Can you work these out from the model? Positions are in its coordinate system, mm. A direction names the side the tool comes from. Coordinates: 2 decimals unless noted, no trailing zeros. Write each loop counter-clockwise with the first axis right and the second up, starting at its lowest first coordinate (ties: lowest second). Pieces come first, ordered by that corner, then holes. Notation, with made-up numbers: M -12.75,-23 L 6.25,-23 A23 cw 6.25,5 Z; hole C 18,86.25 d5. An arc over 180 degrees is marked long. Answer as a JSON object with one key per item and string values. Group by question number.
from build123d import *

# Parameters (mm, degrees)
SKETCH1_W           = 25
SKETCH1_H           = 50
BOSS_EXTRUDE1_DEPTH = 30
SKETCH2_W           = 50
SKETCH2_H           = 8.605036789
BOSS_EXTRUDE2_DEPTH = 20
SKETCH3_R           = 4
CUT_EXTRUDE1_DEPTH  = 47.249264327
SKETCH4_W           = 10.2
SKETCH4_H           = 20.2
CUT_EXTRUDE2_DEPTH  = 20
BOSS_EXTRUDE3_DEPTH = 1


with BuildPart() as part:
    # Sketch1 → Boss-Extrude1 (new body)
    with BuildSketch(Plane(origin=(0, 0, 0), x_dir=(1, 0, 0), z_dir=(0, 1, 0))):
        Rectangle(SKETCH1_W, SKETCH1_H)
    extrude(amount=BOSS_EXTRUDE1_DEPTH)

    # Sketch2 → Boss-Extrude2 (add)
    with BuildSketch(Plane.ZY.offset(12.5)):
        with Locations((0, 4.302518394)):
            Rectangle(SKETCH2_W, SKETCH2_H)
    extrude(amount=BOSS_EXTRUDE2_DEPTH)

    # Sketch3 → Cut-Extrude1 (cut, through all)
    with BuildSketch(Plane(origin=(0, 8.605036789, 0), x_dir=(1, 0, 0), z_dir=(0, 1, 0))):
        with Locations(Location((-24.5, 15, 0), (0, 0, 270))):
            Circle(SKETCH3_R)
        with Locations(Location((-24.5, -15, 0), (0, 0, 270))):
            Circle(SKETCH3_R)
    extrude(amount=-CUT_EXTRUDE1_DEPTH, mode=Mode.SUBTRACT)

    # Sketch4 → Cut-Extrude2 (cut)
    with BuildSketch(Plane(origin=(12.5, 0, 0), x_dir=(0, 0, -1), z_dir=(1, 0, 0))):
        with Locations((15, 15)):
            Rectangle(SKETCH4_W, SKETCH4_H)
    extrude(amount=-CUT_EXTRUDE2_DEPTH, mode=Mode.SUBTRACT)

    # Sketch5 → Boss-Extrude3 (add)
    with BuildSketch(Plane(origin=(0, 30, 0), x_dir=(1, 0, 0), z_dir=(0, 1, 0))):
        with BuildLine():
            Line((7.692307692, 10), (7.692307692, -10))
            Line((7.692307692, -10), (-0.985576923, -10))
            add(Edge.make_bspline(
                [(-0.985576923, -10), (-1.189915508, -9.998406517), (-1.585388921, -9.995322517), (-2.158891161, -9.97328499), (-2.692933181, -9.926466249), (-3.190880742, -9.87417544), (-3.651881782, -9.796967041), (-4.076156001, -9.706387661), (-4.462076213, -9.599333368), (-4.812578849, -9.472790754), (-5.13779529, -9.329673653), (-5.439160579, -9.1529927), (-5.729614752, -8.959721513), (-5.997579665, -8.730765608), (-6.255124362, -8.484777239), (-6.491466209, -8.20944831), (-6.713599726, -7.911670049), (-6.98368474, -7.480457665), (-7.26734754, -6.902448182), (-7.511671117, -6.168093018), (-7.667028651, -5.399134972), (-7.683798939, -4.873873893), (-7.692307692, -4.607371795)],
                knots=[0, 0, 0, 0, 1.242075696, 2.40389213, 3.487198984, 4.500157661, 5.446319301, 6.326791195, 7.136300648, 7.878370406, 8.590488565, 9.292260633, 9.999224673, 10.708050372, 11.431369221, 12.162165018, 12.910600795, 13.687589445, 15.252257874, 16.810406251, 18.381693487, 20, 20, 20, 20], degree=3))
            add(Edge.make_bspline(
                [(-7.692307692, -4.607371795), (-7.688394011, -4.436288612), (-7.680664221, -4.098387595), (-7.621454116, -3.601582104), (-7.51431592, -3.126906532), (-7.376939813, -2.670193942), (-7.1888858, -2.237951011), (-6.971132957, -1.821215885), (-6.700987613, -1.431932834), (-6.399355855, -1.057091635), (-6.048612719, -0.71360816), (-5.658467411, -0.39614679), (-5.217190586, -0.123711561), (-4.739255324, 0.129469087), (-4.212344466, 0.337396306), (-3.644404331, 0.520482963), (-3.031039376, 0.661647942), (-2.605906991, 0.732754289), (-2.387820513, 0.769230769)],
                knots=[0, 0, 0, 0, 0.982645791, 1.940792824, 2.867691729, 3.775150443, 4.675643875, 5.571354211, 6.471357401, 7.392684514, 8.331098131, 9.285922955, 10.275520706, 11.304845665, 12.388884831, 13.524255008, 14.729980297, 16, 16, 16, 16], degree=3))
            add(Edge.make_bspline(
                [(-2.387820513, 0.769230769), (-2.549345996, 0.849743746), (-2.855664626, 1.002429402), (-3.272498706, 1.255059029), (-3.637663897, 1.492888205), (-3.845092801, 1.671226556), (-3.942307692, 1.754807692)],
                knots=[0, 0, 0, 0, 1.172551213, 2.223638478, 3.167479604, 4, 4, 4, 4], degree=3))
            add(Edge.make_bspline(
                [(-3.942307692, 1.754807692), (-4.131560958, 1.939760877), (-4.519688241, 2.319069404), (-5.049338611, 2.971134565), (-5.573421338, 3.688219618), (-5.888069662, 4.2107727), (-6.049679487, 4.479166667)],
                knots=[0, 0, 0, 0, 0.918170575, 1.883016652, 2.912673989, 4, 4, 4, 4], degree=3))
            Line((-6.049679487, 4.479166667), (-9.330929487, 10))
            Line((-9.330929487, 10), (-6.09775641, 10))
            Line((-6.09775641, 10), (-3.605769231, 5.77724359))
            add(Edge.make_bspline(
                [(-3.605769231, 5.77724359), (-3.516164402, 5.629086783), (-3.342524957, 5.34198322), (-3.091798881, 4.922621923), (-2.845639404, 4.536751784), (-2.618440056, 4.172360633), (-2.395792195, 3.839058208), (-2.196203285, 3.524230537), (-1.99576396, 3.245712753), (-1.765615132, 2.91110533), (-1.484546035, 2.549334189), (-1.156558274, 2.177690005), (-0.854995349, 1.869836465), (-0.473923576, 1.576103263), (-8.0808e-05, 1.307161834), (0.399436219, 1.179583217), (0.592948718, 1.117788462)],
                knots=[0, 0, 0, 0, 1.130591283, 2.190900266, 3.190104209, 4.119071823, 4.994606968, 5.807262858, 6.55236009, 7.234593472, 8.459046683, 9.540234366, 10.471327768, 11.266723835, 12.676093724, 14, 14, 14, 14], degree=3))
            add(Edge.make_bspline(
                [(0.592948718, 1.117788462), (0.674242958, 1.103128347), (0.859840146, 1.069658866), (1.174983707, 1.047799895), (1.556818794, 1.024599522), (1.833541189, 1.025275503), (1.983173077, 1.025641026)],
                knots=[0, 0, 0, 0, 0.709978628, 1.620902492, 2.713552433, 4, 4, 4, 4], degree=3))
            Line((1.983173077, 1.025641026), (4.871794872, 1.025641026))
            Line((4.871794872, 1.025641026), (4.871794872, 10))
            Line((4.871794872, 10), (7.692307692, 10))
        make_face()
        with BuildLine():
            Line((4.871794872, -1.282051282), (-0.484775641, -1.282051282))
            add(Edge.make_bspline(
                [(-0.484775641, -1.282051282), (-0.753386517, -1.286217416), (-1.255529355, -1.294005613), (-1.957518176, -1.361528247), (-2.558000395, -1.467075801), (-3.064646298, -1.627384754), (-3.490432782, -1.842070076), (-3.859462924, -2.104609449), (-4.169752828, -2.430321342), (-4.424939479, -2.80379836), (-4.624425797, -3.210810832), (-4.763816724, -3.641583566), (-4.857398907, -4.087856282), (-4.866967535, -4.393220511), (-4.871794872, -4.547275641)],
                knots=[0, 0, 0, 0, 1.546056516, 2.890207646, 4.055830773, 5.050253158, 5.937355789, 6.790906573, 7.644595853, 8.512568064, 9.38593768, 10.244184789, 11.114197691, 12, 12, 12, 12], degree=3))
            add(Edge.make_bspline(
                [(-4.871794872, -4.547275641), (-4.868088958, -4.659544766), (-4.86083016, -4.879447), (-4.822372143, -5.202097101), (-4.749202425, -5.50786025), (-4.648165007, -5.798940542), (-4.520236894, -6.075969951), (-4.363033481, -6.337858904), (-4.177365929, -6.583269781), (-3.964383478, -6.81341075), (-3.719926868, -7.02284832), (-3.440676061, -7.203538998), (-3.128860999, -7.357089463), (-2.784111469, -7.478956731), (-2.407515729, -7.576430897), (-1.996929252, -7.641277267), (-1.554229928, -7.688199899), (-1.24746496, -7.690912847), (-1.08974359, -7.692307692)],
                knots=[0, 0, 0, 0, 0.965235723, 1.89061323, 2.787065514, 3.661873922, 4.534873316, 5.404925039, 6.281839248, 7.175200054, 8.095223355, 9.040740021, 10.02630299, 11.075573487, 12.177989335, 13.364883635, 14.645170704, 16, 16, 16, 16], degree=3))
            Line((-1.08974359, -7.692307692), (4.871794872, -7.692307692))
            Line((4.871794872, -7.692307692), (4.871794872, -1.282051282))
        make_face(mode=Mode.SUBTRACT)
    extrude(amount=BOSS_EXTRUDE3_DEPTH)


solid = part.part
Q1. If we section it at A-A on x = -24.5: List the corners of the cut face in (y, z) for me.
Q2. If we section it at C-C on y = 6: List the corners of the cut face in (x, z) for me.
Q3. If we section it at B-B on z = -15: List the corners of the cut face in (x, y) for me.
Q4. Will these pins go through, and if not, where does the flat tip stop? pin 1 (2 mm diameter, centred on y = 21, z = -14, fed in from -X); pin 2 (0.5 mm diameter, centred on y = 30.5, z = -6, fed in from -X); pin 3 (10.5 mm diameter, centred on x = -24.5, z = 15, fed in from +Y).
Q5. On a 3-axis mill with a long thin cutter (end or side, diameter ignored), from which of +Z, -Z, +X, -X, +Y, -Y can I reach the whole of each face in a straight line? I mean faces 1 (the flat face through (-22, 8.605, 0)), 2 (the cylindrical face through (-21.8, 4.36, -17.95)), 3 (the flat face through (-32.5, 4, 0)), 4 (the flat face through (3, 15, -20.1)), 5 (the flat face through (0, 30, -6)). Say none if no direction works.
Q6. Please list where these lines run through material, in increasing order: L1, parallel to Z at x = 2.5, y = 15; L2, parallel to Y at x = 3, z = -12.5; L3, parallel to Z at x = -24, y = 2.
Q7. We'd pull the mould along X, two halves only. Please class faces 6 (the flat face through (-12.5, 19, 0)), 7 (the cylindrical face through (-21.8, 4.36, 12.05)), 8 (the flat face through (12.5, 15, 0)), 9 (the flat face through (-4.87, 30.49, -7.92)): pulls with the +X half, pulls with the -X half, needs draft (parallel to the pull), parting line crosses it, or undercut.
Q8. If we section it at D-D on x = 4: List the corners of the cut face in (y, z) for me.
Reply:
{
 "1": {"outline": "M 0,-25 L 8.61,-25 L 8.61,-19 L 0,-19 Z; M 0,-11 L 8.61,-11 L 8.61,11 L 0,11 Z; M 0,19 L 8.61,19 L 8.61,25 L 0,25 Z"},
 "2": {"outline": "M -32.5,-25 L 12.5,-25 L 12.5,-20.1 L -7.5,-20.1 L -7.5,-9.9 L 12.5,-9.9 L 12.5,25 L -32.5,25 Z; hole C -24.5,-15 d8; hole C -24.5,15 d8"},
 "3": {"outline": "M -32.5,0 L -28.5,0 L -28.5,8.61 L -32.5,8.61 Z; M -20.5,0 L 12.5,0 L 12.5,4.9 L -7.5,4.9 L -7.5,25.1 L 12.5,25.1 L 12.5,30 L -12.5,30 L -12.5,8.61 L -20.5,8.61 Z"},
 "4": {"pin 1": "x = -12.5", "pin 2": "x = -7.1", "pin 3": "y = 8.61"},
 "5": {"face 1": "+Z, -Z, -X, +Y", "face 2": "+Y, -Y", "face 3": "+Z, -Z, -X, +Y, -Y", "face 4": "+X", "face 5": "+Y"},
 "6": {"L1": "-25 to -20.1, -9.9 to 25", "L2": "0 to 4.9, 25.1 to 30", "L3": "-25 to -18.97, -11.03 to 11.03, 18.97 to 25"},
 "7": {"face 6": "pulls with the -X half", "face 7": "undercut", "face 8": "pulls with the +X half", "face 9": "undercut"},
 "8": {"outline": "M 0,-25 L 30,-25 L 30,-1.03 L 31,-1.03 L 31,1.28 L 30,1.28 L 30,7.69 L 31,7.69 L 31,10 L 30,10 L 30,25 L 0,25 Z; hole M 4.9,-20.1 L 25.1,-20.1 L 25.1,-9.9 L 4.9,-9.9 Z"}
}
